Check sheet for the modelled part. Datum: model origin and axes. Units: mm. A direction names the side the tool comes from. Give positions to 0.01 mm unless a question says otherwise; leave off trailing zeros. Order: outer loops, then holes, each group sorted by start corner. A loop starts at its lowest first (then second) coordinate and runs counter-clockwise, first axis right, second up.
Item 1: Gauge pin test, flat ends, axial feed: P1, Ø10, axis at y = 10.5, z = -10.5, coming from the +X side; P2, Ø3.5, axis at x = -17.84, y = 11.39, coming from the +Z side; P3, Ø5, axis at x = 10, y = 8, coming from the -Z side; P4, Ø1.4, axis at x = 3.93, y = -30.22, coming from the -Z side. Record the tip position at first contact, or that the pin passes through.
Item 2: Sectioned sample at B-B on x = -0.5. Record the boundary of the cut face in (y, z) (3 decimals).
Item 3: Sectioned sample at A-A on y = 1.27. Record the boundary of the cut face in (x, z) (3 decimals), and give its area (3 significant figures).
Item 4: Material ranges on line 1 along X through (y, z) = (26.5, -8); line 2 along X through (y, z) = (1, -10.5); line 3 along Z through (x, y) = (-16.5, 6), recorded low to high.
Item 5: Release check for a two-part mould opening along X. For faces 1 (the flat face through (19.05, -30, -1)), 2 (the flat face through (-2, -31.75, -1)), 3 (the cylindrical face through (-16.87, 11.69, -7.51)) record: released by +X, released by -X, zero draft, split by the parting line, or undercut.
Item 6: Sectioned sample at C-C on z = -3.5. Record the boundary of the cut face in (x, y) (3 decimals), and give its area (3 significant figures).
Item 7: Access from +Z, -Z, +X, -X, +Y, -Y to the whole of each face (thin tool, end or side, straight path). Record for faces 4 (the flat face through (-6, 8, -2.54)), 5 (the flat face through (-14, 0, 0)), 6 (the flat face through (-18, -30, -12.7)), 7 (the flat face through (18, -29.21, -1)).
Item 8: Sectioned sample at D-D on y = -21. Record the boundary of the cut face in (x, z) (3 decimals).
from build123d import *

# Parameters (mm, degrees)
SKETCH1_W             = 2.437632846
SKETCH1_H             = 63.5
SKETCH1_R             = 1.016
BOSS_EXTRUDE1_DEPTH   = 15.24
BOSS_EXTRUDE1_2_DEPTH = 15.24
SKETCH2_W             = 33.244360662
SKETCH2_H             = 63.5
BOSS_EXTRUDE2_DEPTH   = 2.54
SKETCH3_W             = 38.1
SKETCH3_H             = 12.7
BOSS_EXTRUDE3_DEPTH   = 2.54
SKETCH5_R             = 1.071714946
CUT_EXTRUDE2_DEPTH    = 41.040262237
SKETCH6_R             = 1.016
CUT_EXTRUDE3_DEPTH    = 41.040262237
SKETCH7_W             = 38.1
SKETCH7_H             = 2.54
SKETCH7_R             = 1.071714946
BOSS_EXTRUDE5_DEPTH   = 2.54
CUT_EXTRUDE4_DEPTH    = 41.040262237
BOSS_EXTRUDE6_START   = 4.445
SKETCH9_W             = 25.4
SKETCH9_H             = 63.5
SKETCH9_R             = 11.0000034
BOSS_EXTRUDE6_DEPTH   = 4.445
SKETCH10_W            = 35.662367154
SKETCH10_H            = 2.54
CUT_EXTRUDE5_DEPTH    = 12.7
SKETCH11_R            = 0.889
CUT_EXTRUDE7_DEPTH    = 12.7


with BuildPart() as part:
    # Sketch1 → Boss-Extrude1 (new body)
    with BuildSketch(Plane.XY):
        with Locations((-17.831183577, 0)):
            Rectangle(SKETCH1_W, SKETCH1_H)
        with Locations((-17.840996754, -26.657844962)):
            Circle(SKETCH1_R, mode=Mode.SUBTRACT)
        with Locations((-17.840996754, -11.385809707)):
            Circle(SKETCH1_R, mode=Mode.SUBTRACT)
        with Locations((-17.840996754, 11.385809707)):
            Circle(SKETCH1_R, mode=Mode.SUBTRACT)
        with Locations((-17.840996754, 26.657844962)):
            Circle(SKETCH1_R, mode=Mode.SUBTRACT)
    extrude(amount=-BOSS_EXTRUDE1_DEPTH)

    # Sketch2 → Boss-Extrude2 (add)
    with BuildSketch(Plane.XY):
        with Locations((0.009813177, 0)):
            Rectangle(SKETCH2_W, SKETCH2_H)
    extrude(amount=-BOSS_EXTRUDE2_DEPTH)

    # Sketch3 → Boss-Extrude3 (add)
    with BuildSketch(Plane.XZ.offset(31.75)):
        with Locations((0, -6.35)):
            Rectangle(SKETCH3_W, SKETCH3_H)
    extrude(amount=-BOSS_EXTRUDE3_DEPTH)

    # Sketch5 → Cut-Extrude2 (cut, through all)
    with BuildSketch(Plane.XY):
        with Locations((-17.827792249, -30.48)):
            Circle(SKETCH5_R)
        with Locations((17.827792249, -30.48)):
            Circle(SKETCH5_R)
    extrude(amount=-CUT_EXTRUDE2_DEPTH, mode=Mode.SUBTRACT)

    # Sketch7 → Boss-Extrude5 (add)
    with BuildSketch(Plane(origin=(0, 0, -12.7), x_dir=(-1, 0, 0), z_dir=(0, 0, -1))):
        with Locations((0, -30.48)):
            Rectangle(SKETCH7_W, SKETCH7_H)
        with Locations(Location((-17.827792249, -30.48, 0), (0, 0, 180))):
            Circle(SKETCH7_R, mode=Mode.SUBTRACT)
    extrude(amount=BOSS_EXTRUDE5_DEPTH)

    # Sketch8 → Cut-Extrude4 (cut, through all)
    with BuildSketch(Plane.XY):
        with BuildLine():
            ThreePointArc((-7.068009892, 1.27), (3.931993508, -9.7300034), (14.931996908, 1.27))
            Line((14.931996908, 1.27), (-7.068009892, 1.27))
        make_face()
        with BuildLine():
            Line((-7.068009892, 1.27), (14.931996908, 1.27))
            ThreePointArc((14.931996908, 1.27), (3.931993508, 12.2700034), (-7.068009892, 1.27))
        make_face()
    extrude(amount=-CUT_EXTRUDE4_DEPTH, mode=Mode.SUBTRACT)

    # Sketch9 → Boss-Extrude6 (add)
    with BuildSketch(Plane.XY.offset(BOSS_EXTRUDE6_START)):
        with Locations((3.931993508, 0)):
            Rectangle(SKETCH9_W, SKETCH9_H)
        with Locations((3.931993508, 1.27)):
            Circle(SKETCH9_R, mode=Mode.SUBTRACT)
    extrude(amount=-BOSS_EXTRUDE6_DEPTH)

    # Sketch10 → Cut-Extrude5 (cut)
    with BuildSketch(Plane(origin=(0, 0, -15.24), x_dir=(-1, 0, 0), z_dir=(0, 0, -1))):
        with Locations((-1.218816423, -30.48)):
            Rectangle(SKETCH10_W, SKETCH10_H)
    extrude(amount=-CUT_EXTRUDE5_DEPTH, mode=Mode.SUBTRACT)

    # Sketch11 → Cut-Extrude7 (cut)
    with BuildSketch(Plane.XY.offset(4.445)):
        with Locations((3.931993508, -30.217851705)):
            Circle(SKETCH11_R)
    extrude(amount=-CUT_EXTRUDE7_DEPTH, mode=Mode.SUBTRACT)


with BuildPart() as body_2:
    # Sketch1 → Boss-Extrude1 2 (new body)
    with BuildSketch(Plane.XY):
        with Locations((17.840996754, -26.657844962)):
            Circle(SKETCH1_R)
    extrude(amount=-BOSS_EXTRUDE1_2_DEPTH)

    # Sketch6 → Cut-Extrude3 (cut, through all)
    with BuildSketch(Plane.XY):
        with Locations((17.840996754, -26.657844962)):
            Circle(SKETCH6_R)
    extrude(amount=-CUT_EXTRUDE3_DEPTH, mode=Mode.SUBTRACT)


solid = part.part
Report:
1. P1: stops at x = -16.61
1. P2: stops at z = 0
1. P3: stops at z = -2.54
1. P4: passes through
2. outline: (-31.75, -2.54) - (-8.798, -2.54) - (-8.798, 4.445) - (-31.75, 4.445) - close; (11.338, -2.54) - (31.75, -2.54) - (31.75, 4.445) - (11.338, 4.445) - close
3. outline: (-19.05, -15.24) - (-16.612, -15.24) - (-16.612, -2.54) - (-7.068, -2.54) - (-7.068, 4.445) - (-8.768, 4.445) - (-8.768, 0) - (-19.05, 0) - close; (14.932, -2.54) - (16.632, -2.54) - (16.632, 4.445) - (14.932, 4.445) - close
3. area: 80.8 mm2
4. line 1: x = -19.05 to -18.84, -16.84 to -16.61
4. line 2: x = -19.05 to -16.61
4. line 3: z = -2.54 to 0
5. face 1: released by +X
5. face 2: zero draft
5. face 3: undercut
6. outline: (-19.05, -31.75) - (-16.612, -31.75) - (-16.612, 31.75) - (-19.05, 31.75) - close; hole circle Ø2.143 at (-17.828, -30.48); hole circle Ø2.032 at (-17.841, -26.658); hole circle Ø2.032 at (-17.841, -11.386); hole circle Ø2.032 at (-17.841, 11.386); hole circle Ø2.032 at (-17.841, 26.658)
6. area: 138 mm2
7. face 4: -Z, +X, +Y, -Y
7. face 5: +Z, -X, +Y, -Y
7. face 6: +Z
7. face 7: +Z, -Z, +X, +Y
8. outline: (-19.05, -15.24) - (-16.612, -15.24) - (-16.612, -2.54) - (16.632, -2.54) - (16.632, 4.445) - (-8.768, 4.445) - (-8.768, 0) - (-19.05, 0) - close
